Source: three-view drawing plus pictorial views. Frame: mm from the lowest corner of the part. Round coordinates to 2 decimals unless told otherwise and drop trailing zeros. Loops run counter-clockwise (first coordinate to the right, second up) from the corner with the lowest first, then second, coordinate; pieces in that order, holes last. Notation, with made-up numbers: (55, 63) -> (101, 63) arc R28 cw to (101, 92) -> close; hole circle Ø1 at (39, 37). An arc over 180 degrees is marked (long way). Answer as a JSON object with one key per item and string values. Group by question number.
Item 1: Section query C-C on y = 0.9. Return loops of the section in (x, z).
Item 2: Material intervals for line 1 (Y direction, x = 54, z = 1.95); line 2 (Z direction, x = 54, y = 1.15); line 3 (X direction, y = 1.85, z = 10.25), sorted ascending. Write a range as [from, to].
Item 3: Section query B-B on y = 5.25. Return loops of the section in (x, z).
Item 4: Section query A-A on z = 9.75. Return loops of the section in (x, y).
Item 5: Draft query along Z for the marked faces 1, 2 and 3. Return one class per face: released by +Z, released by -Z, zero draft, split by the parting line, or undercut.
Item 6: Pin query (flat end, axial travel): pin 1 (2.5 mm diameter, centred on x = 54, y = 3, fed in from -Z); pin 2 (0.9 mm diameter, centred on y = 3.5, z = 1, fed in from -X); pin 3 (6 mm diameter, centred on x = 28.5, z = 9, fed in from -Y); pin 4 (1.8 mm diameter, centred on x = 2, y = 2.5, fed in from +Z). Return the tip coordinate at first contact, or that it passes through.
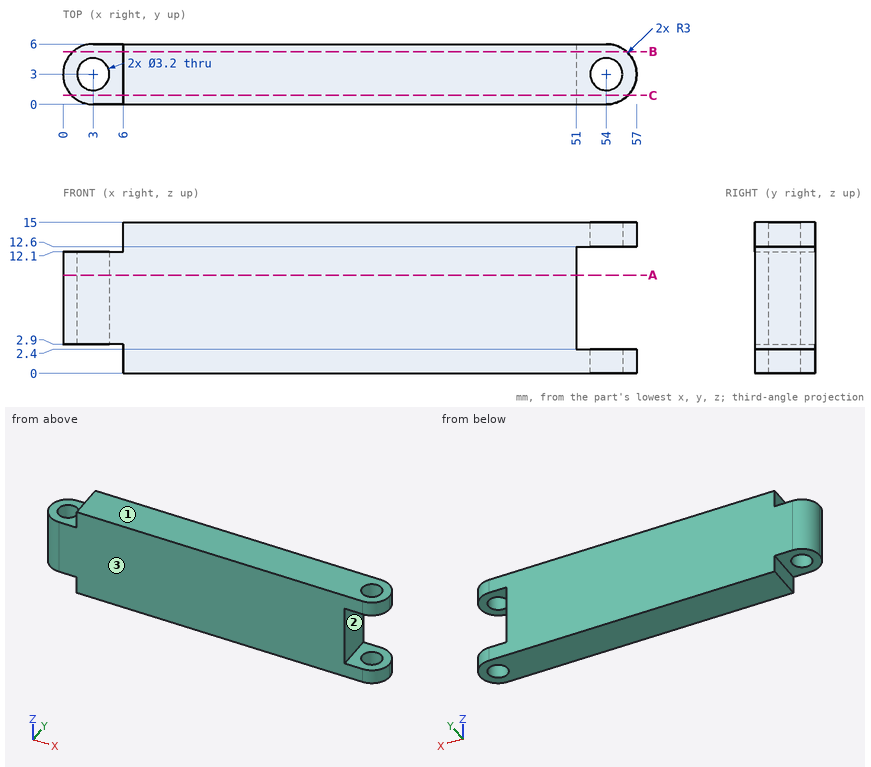
Solved:
{
 "1": {"outline": "(0.86, 2.9) -> (6, 2.9) -> (6, 0) -> (56.14, 0) -> (56.14, 2.4) -> (51, 2.4) -> (51, 12.6) -> (56.14, 12.6) -> (56.14, 15) -> (6, 15) -> (6, 12.1) -> (0.86, 12.1) -> close"},
 "2": {"line 1": "[0, 1.4], [4.6, 6]", "line 2": "[0, 2.4], [12.6, 15]", "line 3": "[0.23, 1.89], [4.11, 51]"},
 "3": {"outline": "(1.02, 2.9) -> (6, 2.9) -> (6, 0) -> (55.98, 0) -> (55.98, 2.4) -> (51, 2.4) -> (51, 12.6) -> (55.98, 12.6) -> (55.98, 15) -> (6, 15) -> (6, 12.1) -> (1.02, 12.1) -> close"},
 "4": {"outline": "(3, 0) -> (51, 0) -> (51, 6) -> (3, 6) arc R3 ccw to start; hole circle Ø3.2 at (3, 3)"},
 "5": {"face 1": "released by +Z", "face 2": "undercut", "face 3": "zero draft"},
 "6": {"pin 1": "through", "pin 2": "x = 6", "pin 3": "y = 0", "pin 4": "z = 12.1"}
}
